Design review of the part built by this model. Coordinates are the model's own, in mm. Face numbers are marked on the shaded views. A direction names the side the tool comes from. Coordinates: 2 decimals unless noted, no trailing zeros. Loops run counter-clockwise (first coordinate to the right, second up) from the corner with the lowest first, then second, coordinate; pieces in that order, holes last. Notation, with made-up numbers: (3, -17.75) -> (38, -17.75) arc R16 cw to (38, -6.75) -> close; hole circle Ø5 at (71, -33.5). An arc over 180 degrees is marked (long way). Answer as a JSON object with one key per item and string values.
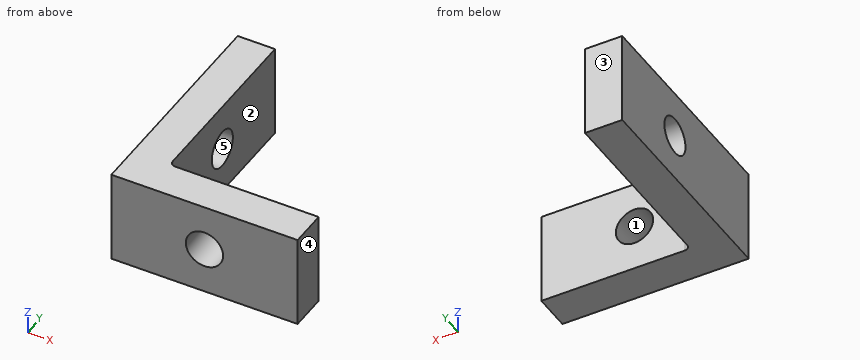
```python
from build123d import *

# Parameters (mm, degrees)
SKETCH1_W           = 100
SKETCH1_H           = 50
BOSS_EXTRUDE1_DEPTH = 20
SKETCH3_W           = 20
SKETCH3_H           = 50
BOSS_EXTRUDE2_DEPTH = 100
SKETCH4_R           = 10
CUT_EXTRUDE1_DEPTH  = 100
SKETCH5_R           = 10
CUT_EXTRUDE2_DEPTH  = 100
FILLET1_R           = 3


with BuildPart() as part:
    # Sketch1 → Boss-Extrude1 (new body)
    with BuildSketch(Plane(origin=(0, 0, 0), x_dir=(1, 0, 0), z_dir=(0, 1, 0))):
        Rectangle(SKETCH1_W, SKETCH1_H)
    extrude(amount=BOSS_EXTRUDE1_DEPTH)

    # Sketch3 → Boss-Extrude2 (add)
    with BuildSketch(Plane(origin=(0, 20, 0), x_dir=(1, 0, 0), z_dir=(0, 1, 0))):
        with Locations((-40, 0)):
            Rectangle(SKETCH3_W, SKETCH3_H)
    extrude(amount=BOSS_EXTRUDE2_DEPTH)

    # Sketch4 → Cut-Extrude1 (cut)
    with BuildSketch(Plane(origin=(-30, 0, 0), x_dir=(0, 0, -1), z_dir=(1, 0, 0))):
        with Locations((0, 70)):
            Circle(SKETCH4_R)
    extrude(amount=-CUT_EXTRUDE1_DEPTH, mode=Mode.SUBTRACT)

    # Sketch5 → Cut-Extrude2 (cut)
    with BuildSketch(Plane(origin=(0, 20, 0), x_dir=(1, 0, 0), z_dir=(0, 1, 0))):
        with Locations(Location((0, 0, 0), (0, 0, 270))):
            Circle(SKETCH5_R)
    extrude(amount=-CUT_EXTRUDE2_DEPTH, mode=Mode.SUBTRACT)

    # Fillet1
    fillet1_edges = [part.edges().sort_by_distance(p)[0] for p in [
        (-30, 20, 0),
    ]]
    fillet(fillet1_edges, radius=FILLET1_R)


solid = part.part
```
1) For the marked faces 1 and 2, list the 3-axis set-ups (+Z, -Z, +X, -X, +Y, -Y) from which the entire face can be reached by the end or side of a thin tool; tool diameter is ignored.
Completed:
{"face 1": "+Y, -Y", "face 2": "+Z, -Z, +X, +Y"}
2) Add section D-D, the plane x = -36.5. Give the boundary of the cut face in (y, z), and give its area (3 significant figures).
Completed:
{"outline": "(0, -25) -> (120, -25) -> (120, 25) -> (0, 25) -> close; hole circle Ø20 at (70, 0)", "area": "5,690 mm²"}
3) The part is to be moulded in two halves that separate along Y. For the marked faces 3, 4 and 5, say which applies: pulls with the +Y half, pulls with the -Y half, needs draft (parallel to the pull), parting line crosses it, or undercut.
Completed:
{"face 3": "pulls with the +Y half", "face 4": "needs draft", "face 5": "undercut"}
4) Add section B-B, the plane y = 70. Give the boundary of the cut face in (x, z).
Completed:
{"outline": "(-50, -25) -> (-30, -25) -> (-30, -10) -> (-50, -10) -> close; (-50, 10) -> (-30, 10) -> (-30, 25) -> (-50, 25) -> close"}
5) Add section A-A, the plane x = 0. Give the boundary of the cut face in (y, z), and give its area (3 significant figures).
Completed:
{"outline": "(0, -25) -> (20, -25) -> (20, -10) -> (0, -10) -> close; (0, 10) -> (20, 10) -> (20, 25) -> (0, 25) -> close", "area": "600 mm²"}
6) Wall thickness on probe 1 along Y at (x, z) = (-31, -0.5); probe 2 along X at (y, z) = (6, 0); probe 3 along X at (y, z) = (37, 1): over which ranges is each line inside the solid? List them lowest first.
Completed:
{"probe 1": "0 to 60.01, 79.99 to 120", "probe 2": "-50 to -10, 10 to 50", "probe 3": "-50 to -30"}
7) Clearance check with flat-ended pins moving along their axes: pin 1 Ø5 at (x, z) = (24, -3) entering from -Y; pin 2 Ø1.5 at (x, z) = (-2, -8.5) entering from +Y; pin 3 Ø10 at (y, z) = (57, 0.5) entering from +X; pin 4 Ø10 at (x, z) = (5, -9) entering from +Y. State where each tip first meets the part, or that it passes through.
Completed:
{"pin 1": "y = 0", "pin 2": "through", "pin 3": "x = -30", "pin 4": "y = 20"}
8) Add section C-C, the plane z = 0. Give the boundary of the cut face in (x, y).
Completed:
{"outline": "(-50, 0) -> (-10, 0) -> (-10, 20) -> (-27, 20) arc R3 cw to (-30, 23) -> (-30, 60) -> (-50, 60) -> close; (-50, 80) -> (-30, 80) -> (-30, 120) -> (-50, 120) -> close; (10, 0) -> (50, 0) -> (50, 20) -> (10, 20) -> close"}
